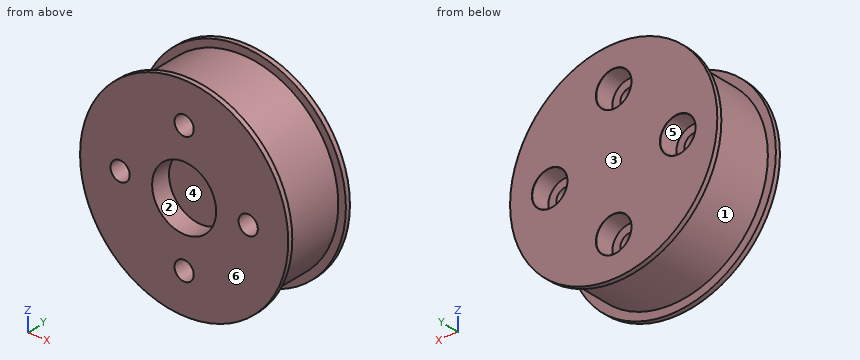
from build123d import *

# Parameters (mm, degrees)
CBORE_FOR_M2_HEX_SOCKET_HEAD_CAP_SCR_2_COUNT = 2
CBORE_FOR_M2_HEX_SOCKET_HEAD_CAP_SCR_2_PITCH = 11.313708499
CBORE_FOR_M2_HEX_SOCKET_HEAD_CAP_SCR_3_COUNT = 2
CBORE_FOR_M2_HEX_SOCKET_HEAD_CAP_SCR_3_PITCH = 16
CBORE_FOR_M2_HEX_SOCKET_HEAD_CAP_SCR_4_COUNT = 2
CBORE_FOR_M2_HEX_SOCKET_HEAD_CAP_SCR_4_PITCH = 11.313708499
SKETCH6_R                                    = 4
CUT_EXTRUDE1_DEPTH                           = 2.5


with BuildPart() as part:
    # Sketch1 → Revolve1 (revolve)
    with BuildSketch(Plane.XY, mode=Mode.PRIVATE) as revolve1_sk:
        Polygon((0, 0), (13, 0), (13, 0.6), (12, 0.6), (12, 8.6), (12.942857143, 8.6), (12.942857143, 9.2), (0, 9.2), align=None)
    revolve(revolve1_sk.sketch.rotate(Axis((0, 9.2, 0), (0, -1, 0)), 180), axis=Axis((0, 9.2, 0), (0, -1, 0)))

    # Sketch3 → CBORE for M2 Hex Socket Head Cap Screw1 (revolve, cut)
    with BuildSketch(Plane(origin=(-8, 9.2, 0), x_dir=(0, 0, 1), z_dir=(1, 0, 0))):
        Polygon((0, 0), (0, 9.2), (1.2, 9.2), (1.2, 2.4), (2.2, 2.4), (2.2, 0.025), (2.225, 0), align=None)
    cbore_for_m2_hex_socket_head_cap_screw1 = revolve(axis=Axis((-8, 15.55, 0), (0, -1, 0)), mode=Mode.SUBTRACT)

    # CBORE for M2 Hex Socket Head Cap Scr 2: CBORE for M2 Hex Socket Head Cap Screw1 ×2
    with Locations(*[Vector(0.7071067811865277, 0, -0.7071067811865673) * (i * CBORE_FOR_M2_HEX_SOCKET_HEAD_CAP_SCR_2_PITCH) for i in range(1, CBORE_FOR_M2_HEX_SOCKET_HEAD_CAP_SCR_2_COUNT)]):
        add(cbore_for_m2_hex_socket_head_cap_screw1, mode=Mode.SUBTRACT)

    # CBORE for M2 Hex Socket Head Cap Scr 3: CBORE for M2 Hex Socket Head Cap Screw1 ×2
    with Locations(*[(i * CBORE_FOR_M2_HEX_SOCKET_HEAD_CAP_SCR_3_PITCH, 0, 0) for i in range(1, CBORE_FOR_M2_HEX_SOCKET_HEAD_CAP_SCR_3_COUNT)]):
        add(cbore_for_m2_hex_socket_head_cap_screw1, mode=Mode.SUBTRACT)

    # CBORE for M2 Hex Socket Head Cap Scr 4: CBORE for M2 Hex Socket Head Cap Screw1 ×2
    with Locations(*[Vector(0.7071067811865674, 0, 0.7071067811865276) * (i * CBORE_FOR_M2_HEX_SOCKET_HEAD_CAP_SCR_4_PITCH) for i in range(1, CBORE_FOR_M2_HEX_SOCKET_HEAD_CAP_SCR_4_COUNT)]):
        add(cbore_for_m2_hex_socket_head_cap_screw1, mode=Mode.SUBTRACT)

    # Sketch6 → Cut-Extrude1 (cut)
    with BuildSketch(Plane.XZ):
        with Locations(Location((0, 0, 0), (0, 0, 270))):
            Circle(SKETCH6_R)
    extrude(amount=-CUT_EXTRUDE1_DEPTH, mode=Mode.SUBTRACT)


solid = part.part
Model file for the job. Use its own axes, mm. Face numbers are marked on the shaded views. A direction names the side the tool comes from. Give positions to 0.01 mm unless a question says otherwise; leave off trailing zeros. Loops run counter-clockwise (first coordinate to the right, second up) from the corner with the lowest first, then second, coordinate; pieces in that order, holes last.
1) Tool access for the marked faces 4, 5 and 6: list every direction of +Z, -Z, +X, -X, +Y, -Y with a clear straight run to the whole face (end or side of a thin tool).
2) Flat gauge pins, fed straight in: pin 1 Ø1 at (x, z) = (4.5, -7.5) entering from -Y; pin 2 Ø2.5 at (x, z) = (0, -8) entering from +Y; pin 3 Ø4 at (x, y) = (3.5, 8) entering from -Z; pin 4 Ø2 at (y, z) = (6, 3) entering from -X. Where does each tip first touch, or does it go through?
3) Saw through at D-D (y = 8). Write the cut outline in (x, z), plus the area to 3 significant figures.
4) Saw through at B-B (y = 1). Write the cut outline in (x, z), plus the area to 3 significant figures.
5) Saw through at C-C (x = -8). Write the cut outline in (y, z) (3 decimals), plus the area to 3 significant figures.
6) Saw through at A-A (z = -8). Write the cut outline in (x, y) (3 decimals).
7) Wall check: line 1 (Y direction, x = -5.5, z = -11); line 2 (Z direction, x = -1, y = 7); line 3 (X direction, y = 3.5, z = 0.5). Give the ranges that are in metal, low to high.
8) Pull direction Z, two halves, no side cores. Call the marked faces 1, 2 and 3: +Z half, -Z half, draft (parallel to the pull), parting line (faces both ways), or undercut.
Answer block:
1. face 4: -Y
1. face 5: +Y
1. face 6: +Z, -Z, +X, -X, -Y
2. pin 1: stops at y = 0
2. pin 2: stops at y = 6.8
2. pin 3: stops at z = -12.84
2. pin 4: stops at x = -11.83
3. outline: circle Ø24 at (0, 0); hole circle Ø4.4 at (-8, 0); hole circle Ø4.4 at (0, -8); hole circle Ø4.4 at (0, 8); hole circle Ø4.4 at (8, 0)
3. area: 392 mm2
4. outline: circle Ø24 at (0, 0); hole circle Ø2.4 at (-8, 0); hole circle Ø8 at (0, 0); hole circle Ø2.4 at (0, -8); hole circle Ø2.4 at (0, 8); hole circle Ø2.4 at (8, 0)
4. area: 384 mm2
5. outline: (0, -10.247) - (0.6, -10.247) - (0.6, -8.944) - (8.6, -8.944) - (8.6, -10.174) - (9.2, -10.174) - (9.2, -2.225) - (9.175, -2.2) - (6.8, -2.2) - (6.8, -1.2) - (0, -1.2) - close; (0, 1.2) - (6.8, 1.2) - (6.8, 2.2) - (9.175, 2.2) - (9.2, 2.225) - (9.2, 10.174) - (8.6, 10.174) - (8.6, 8.944) - (0.6, 8.944) - (0.6, 10.247) - (0, 10.247) - close
5. area: 141 mm2
6. outline: (-10.247, 0) - (-1.2, 0) - (-1.2, 6.8) - (-2.2, 6.8) - (-2.2, 9.175) - (-2.225, 9.2) - (-10.174, 9.2) - (-10.174, 8.6) - (-8.944, 8.6) - (-8.944, 0.6) - (-10.247, 0.6) - close; (1.2, 0) - (10.247, 0) - (10.247, 0.6) - (8.944, 0.6) - (8.944, 8.6) - (10.174, 8.6) - (10.174, 9.2) - (2.225, 9.2) - (2.2, 9.175) - (2.2, 6.8) - (1.2, 6.8) - close
7. line 1: y = 0 to 0.6, 8.6 to 9.2
7. line 2: z = -11.96 to -9.96, -6.04 to 6.04, 9.96 to 11.96
7. line 3: x = -11.99 to -9.09, -6.91 to 6.91, 9.09 to 11.99
8. face 1: parting line
8. face 2: undercut
8. face 3: draft
